from build123d import *

# Parameters (mm, degrees)
BOX184_W          = 10
BOX184_H          = 3.5
BOX184_DEPTH      = 3
CYLINDER071_R     = 1.6
CYLINDER071_DEPTH = 2
BOX182_W          = 10
BOX182_H          = 2
BOX182_DEPTH      = 12
FILLET041_R       = 3


with BuildPart() as cube173:
    # Box184 → Box184 (new body)
    with BuildSketch(Plane(origin=(30, 29.5, -16), x_dir=(1, 0, 0), z_dir=(0, 0, 1))):
        with Locations((5, 1.75)):
            Rectangle(BOX184_W, BOX184_H)
    extrude(amount=BOX184_DEPTH)


with BuildPart() as cylinder152:
    # Cylinder071 → Cylinder071 (new body)
    with BuildSketch(Plane(origin=(35, 35, -22), x_dir=(1, 0, 0), z_dir=(0, -1, 0))):
        Circle(CYLINDER071_R)
    extrude(amount=CYLINDER071_DEPTH)


with BuildPart() as fusion057:
    # Box182 → Box182 (new body)
    with BuildSketch(Plane(origin=(30, 33, -25), x_dir=(1, 0, 0), z_dir=(0, 0, 1))):
        with Locations((5, 1)):
            Rectangle(BOX182_W, BOX182_H)
    extrude(amount=BOX182_DEPTH)

    # Cut096: cut Cylinder152
    add(cylinder152.part, mode=Mode.SUBTRACT)

    # Fillet041
    fillet041_edges = [fusion057.edges().sort_by_distance(p)[0] for p in [
        (30, 34, -25),
        (40, 34, -25),
    ]]
    fillet(fillet041_edges, radius=FILLET041_R)

    # Fusion057: union Cube173
    add(cube173.part)


solid = fusion057.part
The listing builds one solid part. Answer for the finished solid, in the listing's coordinates (mm). Round coordinates to 2 decimals unless told otherwise and drop trailing zeros. Order: outer loops, then holes, each group sorted by start corner. A loop starts at its lowest first (then second) coordinate and runs counter-clockwise, first axis right, second up. Notation, with made-up numbers: M 44.25,-14.5 L 95.25,-14.5 A22 cw 95.25,-5.5 Z; hole C 57.25,51 d6. An arc over 180 degrees is marked long. Answer in a Markdown table with one row per item. Add a question column.
1) The part is cut by section D-D on y = 31.3. Determine the outline of the cut face in (x, z).
2) Consider line 1 along Z through (x, y) = (35, 34); line 2 along Y through (x, z) = (33.5, -23); line 3 along Z through (x, y) = (33, 30.15). Determine where each line is inside the solid, lowest interval first. Write a range as from..to.
3) Determine the mould class of faces 1 (the face through (35, 33, -20)), 2 (the face through (33.82, 34.01, -20.92)), 3 (the face through (35, 31, -16)) for opening direction Z: pulls with the +Z half, pulls with the -Z half, needs draft (parallel to the pull), parting line crosses it, or undercut.
4) The part is cut by section B-B on x = 33.25. Determine the outline of the cut face in (y, z).
5) The part is cut by section C-C on z = -19.5. Determine the outline of the cut face in (x, y), plus the area to 3 significant figures.
6) Flat-ended cylindrical pins translate along their axes: pin 1 Ø1 at (x, z) = (36, -22) entering from -Y; pin 2 Ø4 at (x, z) = (35, -22) entering from -Y; pin 3 Ø1.8 at (x, y) = (34.5, 31) entering from -Z. Find the tip coordinate at first contact, or state that the pin passes through.
7) The part is cut by section A-A on x = 35. Determine the outline of the cut face in (y, z).
Findings below:
| question | item | result |
|---|---|---|
| 1 | outline | M 30,-16 L 40,-16 L 40,-13 L 30,-13 Z |
| 2 | line 1 | z = -25..-23.6, -20.4..-13 |
| 2 | line 2 | y = 33..35 |
| 2 | line 3 | z = -16..-13 |
| 3 | face 1 | needs draft |
| 3 | face 2 | undercut |
| 3 | face 3 | pulls with the -Z half |
| 4 | outline | M 29.5,-16 L 33,-16 L 33,-25 L 35,-25 L 35,-13 L 29.5,-13 Z |
| 5 | outline | M 30,33 L 40,33 L 40,35 L 30,35 Z |
| 5 | area | 20.0 mm² |
| 6 | pin 1 | passes through |
| 6 | pin 2 | stops at y = 33 |
| 6 | pin 3 | stops at z = -16 |
| 7 | outline | M 29.5,-16 L 33,-16 L 33,-20.4 L 35,-20.4 L 35,-13 L 29.5,-13 Z; M 33,-25 L 35,-25 L 35,-23.6 L 33,-23.6 Z |
